The model under review builds one solid part; all positions refer to its coordinate system, in mm. A direction names the side the tool comes from. Round coordinates to 2 decimals unless told otherwise and drop trailing zeros. Loops run counter-clockwise (first coordinate to the right, second up) from the corner with the lowest first, then second, coordinate; pieces in that order, holes last. Notation, with made-up numbers: M 41,22 L 83,22 A24 ccw 83,32 Z; hole C 19.25,58.5 d9. An arc over 180 degrees is marked long. Return JSON: item names as keys, results as strings. Group by question number.
Q1. For faces 1 (the face through (-4.56, 0.99, 0.91)), 2 (the face through (-1, 1, 3.5)), 3 (the face through (-8, 0.6, 0)), list the 3-axis set-ups (+Z, -Z, +X, -X, +Y, -Y) from which the entire face can be reached by the end or side of a thin tool; tool diameter is ignored.
Q2. Clearance check with flat-ended pins moving along their axes: pin 1 Ø3 at (x, z) = (5, 0) entering from +Y; pin 2 Ø3.5 at (x, z) = (-5.75, 0) entering from +Y; pin 3 Ø1.5 at (x, z) = (5.5, -0.5) entering from +Y. State where each tip first meets the part, or that it passes through.
Q3. To check wall thickness, follow line 1 along X through (y, z) = (0.35, -2.5); line 2 along Z through (x, y) = (-5.75, 0.9); line 3 along X through (y, z) = (1.9, 0). State the ranges of each line that lie inside material, in increasing order.
Q4. Draft analysis for pull direction Z (two halves, no side actions). For faces 4 (the face through (-6, 0.5, 0)), 5 (the face through (-1, 1, -3.5)), 6 (the face through (-9.4, 1, 0)), state which applies: pulls with the +Z half, pulls with the -Z half, needs draft (parallel to the pull), parting line crosses it, or undercut.
Q5. Consider section C-C (x = 0). State the section outline as (y, z) points.
Q6. Consider section A-A (z = 0). State the section outline as (x, y) points, and give its area (3 significant figures).
Q7. Consider section B-B (y = 1.75). State the section outline as (x, z) points, and give its area (3 significant figures).
Q8. Consider section D-D (z = -2.25). State the section outline as (x, y) points.
Autodesk Inventor part; units mm, degrees
ref_plane "YZ Plane" through (0, 0, 0) normal (1, 0, 0) x (0, 1, 0)
ref_plane "XZ Plane" through (0, 0, 0) normal (0, 1, 0) x (-1, 0, 0)
ref_plane "XY Plane" through (0, 0, 0) normal (0, 0, 1) x (1, 0, 0)
sketch "Sketch1" plane through (0, 0, 0) normal (0, 1, 0) x (-1, 0, 0)
  line L0 (-10, 3.5) -> (10, 3.5)
  line L1 (10, 3.5) -> (10, -3.5)
  line L2 (10, -3.5) -> (-10, -3.5)
  line L3 (-10, -3.5) -> (-10, 3.5)
  line L4 (-10, 3.5) -> (10, -3.5) construction
  line L5 (10, 3.5) -> (-10, -3.5) construction
  line L6 (-10, 0) -> (10, 0) construction
  circle A0 centre (-5.75, 0) radius 1.5
  circle A1 centre (5.75, 0) radius 1.5
  circle A2 centre (0, 0) radius 1.5
  line L7 (-8.3, 3.5) -> (-8.3, -3.5)
  point P0 (0, 0)
  dimension "d0" = 7
  dimension "d1" = 20
  dimension "d2" = 3
  dimension "d3" = 3
  dimension "d4" = 3
  dimension "d5" = 5.75
  dimension "d6" = 5.75
  dimension "d7" = 4.25
  dimension "d8" = 4.25
  dimension "d16" = 1.7
extrude "Extrusion1" add sketch "Sketch1" along normal blind 2 contours L0 L1 L2 L7
extrude "Extrusion2" add sketch "Sketch1" along normal blind 0.5 contours A0 | A1 | A2
chamfer "Chamfer1" distance 0.5 angle 45 3 edges at (7.25, 2, 0) (1.5, 2, 0) (-4.25, 2, 0)
sketch "Sketch2" plane through (-10, 0, 3.5) normal (0, 0, 1) x (1, 0, 0)
  line L0 (0, 0) -> (18.3, 0)
  line L1 (18.3, 0) -> (18.3, 2)
  line L2 (0, 2) -> (18.3, 2)
  line L3 (0, 0) -> (0, 2)
  line L4 (2.75, 1.5) -> (5.75, 1.5)
  line L5 (6.25, 2) -> (2.25, 2)
  line L6 (2.75, 1.5) -> (2.25, 2)
  line L7 (2.6, 0) -> (1.4, 1.2)
  line L8 (0.6, 1.2) -> (0.6, 0)
  line L9 (2.75, 0.5) -> (5.75, 0.5)
  line L10 (2.75, 1.5) -> (2.75, 0.5)
  line L11 (2.75, 1.5) -> (2.75, 0.5)
  line L12 (5.75, 0.5) -> (5.75, 1.5)
  line L13 (5.75, 1.5) -> (6.25, 2)
  line L14 (1.4, 1.2) -> (0.6, 1.2)
  point P0 (10, 0)
  dimension "d17" = 0.6
  dimension "d18" = 90
  dimension "d19" = 45
  dimension "d21" = 0.8
  dimension "d22" = 1.2
  dimension "d23" = 0.4596
extrude "Extrusion3" cut sketch "Sketch2" against normal through all contours L8 L14 L7 L0
equation "\"d6\" = d5"
equation "\"d7\" = d5 - 0.5 * d3"
equation "\"d8\" = d5 - 0.5 * d2"
properties part number "glue_test_flex_2"
Values:
{
 "1": {"face 1": "+Y", "face 2": "+Z, +X, -X, +Y, -Y", "face 3": "+Z, -Z, -Y"},
 "2": {"pin 1": "stops at y = 2", "pin 2": "stops at y = 1.75", "pin 3": "stops at y = 0.5"},
 "3": {"line 1": "x = -10 to -9.4, -7.75 to 8.3", "line 2": "z = -3.5 to -1.5, 1.5 to 3.5", "line 3": "x = -10 to -7.65, -3.85 to -1.9, 1.9 to 3.85, 7.65 to 8.3"},
 "4": {"face 4": "undercut", "face 5": "pulls with the -Z half", "face 6": "needs draft"},
 "5": {"outline": "M 0,-3.5 L 2,-3.5 L 2,-2 L 1.5,-1.5 L 0.5,-1.5 L 0.5,1.5 L 1.5,1.5 L 2,2 L 2,3.5 L 0,3.5 Z"},
 "6": {"outline": "M -10,0 L -9.4,0 L -9.4,1.2 L -8.6,1.2 L -7.4,0 L 8.3,0 L 8.3,2 L 7.75,2 L 7.25,1.5 L 7.25,0.5 L 4.25,0.5 L 4.25,1.5 L 3.75,2 L 2,2 L 1.5,1.5 L 1.5,0.5 L -1.5,0.5 L -1.5,1.5 L -2,2 L -3.75,2 L -4.25,1.5 L -4.25,0.5 L -7.25,0.5 L -7.25,1.5 L -7.75,2 L -10,2 Z", "area": "20.7 mm2"},
 "7": {"outline": "M -10,-3.5 L 8.3,-3.5 L 8.3,3.5 L -10,3.5 Z; hole C -5.75,0 d3.5; hole C 0,0 d3.5; hole C 5.75,0 d3.5", "area": "99.2 mm2"},
 "8": {"outline": "M -10,0 L -9.4,0 L -9.4,1.2 L -8.6,1.2 L -7.4,0 L 8.3,0 L 8.3,2 L -10,2 Z"}
}
